```python
from build123d import *

# Parameters (mm, degrees)
CONECUT_DEPTH      = 53.387999569
CONECUT_DEPTH_BACK = 53.387999569


with BuildPart() as part:
    # Body: sweep along a path in PathSke
    with BuildLine(Plane.XY) as body_path:
        Line((45, 4.75), (0, 4.75))
        ThreePointArc((0, 4.75), (-1.846620522, 5.148259898), (-3.364941176, 6.272235294))
        ThreePointArc((-3.364941176, 6.272235294), (-20, 0), (-3.364941176, -6.272235294))
        ThreePointArc((-3.364941176, -6.272235294), (-1.846620522, -5.148259898), (0, -4.75))
        Line((0, -4.75), (51.3, -4.75))
    # SectionSke → Body (sweep)
    with BuildSketch(Plane(origin=(45, 0, 0), x_dir=(0, 0, -1), z_dir=(1, 0, 0))):
        with BuildLine():
            Line((-4.749999579, 0.002), (4.749999579, 0.002))
            ThreePointArc((4.749999579, 0.002), (0, 4.75), (-4.749999579, 0.002))
        make_face()
    sweep(path=body_path.line)

    # ConeCutSke → ConeCut (cut, two sides: drawn at the far end of the back side and taken through both)
    with BuildSketch(Plane.XY.offset(-CONECUT_DEPTH_BACK)):
        Polygon((45, 2.376), (41.603808574, 4.76), (51.31, 4.76), (51.31, -4.76), (47.903808574, -4.76), (51.3, -2.376), (47.898206914, 0), (41.598206914, 0), align=None)
    extrude(amount=CONECUT_DEPTH + CONECUT_DEPTH_BACK, mode=Mode.SUBTRACT)


solid = part.part
```
Design review of the part built by this model. Coordinates are the model's own, in mm. A direction names the side the tool comes from. Round coordinates to 2 decimals unless told otherwise and drop trailing zeros. Order: outer loops, then holes, each group sorted by start corner. A loop starts at its lowest first (then second) coordinate and runs counter-clockwise, first axis right, second up. Notation, with made-up numbers: (88, -27) - (140, -27) arc R26 ccw to (140, 6) - close; hole circle Ø1 at (54, 28). An arc over 180 degrees is marked (long way). Return JSON: item names as keys, results as strings.
Q1. Machinability: for faces 1 (the cylindrical face through (-15.25, 0.16, -0.07)), 2 (the cylindrical face through (26.01, -4.75, 0.1)), 3 (the cylindrical face through (22.18, 4.75, 0.1)), which of the approach directions +Z, -Z, +X, -X, +Y, -Y give a long, thin tool a straight path to every point of the face, cutting with its end or side? Answer none if there is none.
Computed values:
{"face 1": "+Z, -Z", "face 2": "+X, -Y", "face 3": "+X, +Y"}
Q2. Consider section B-B on x = 43.5. Write out the cut boundary in (y, z), plus the area to 3 significant figures.
Computed values:
{"outline": "(0, -4.75) - (0, 4.75) arc R4.75 ccw to start; (1.33, -4.56) arc R4.75 ccw to (3.43, -3.29) - (3.43, 3.29) arc R4.75 ccw to (1.33, 4.56) - close", "area": "52.4 mm2"}
Q3. Consider section A-A on z = 0. Write out the cut boundary in (x, y), plus the area to 3 significant figures.
Computed values:
{"outline": "(-6.93, -3.14) arc R4.75 cw (long way) to (-6.93, 3.14) arc R9.23 ccw to (0, 0) - (41.6, 0) - (45, 2.38) - (41.62, 4.75) - (0, 4.75) arc R4.48 cw to (-3.36, 6.27) arc R9.5 ccw (long way) to (-3.36, -6.27) arc R4.48 cw to (0, -4.75) - (47.92, -4.75) - (51.3, -2.38) - (47.9, 0) - (0, 0) arc R9.23 ccw to start", "area": "660 mm2"}
Q4. For pin 1 Ø1 at (x, y) = (-0.5, -2) entering from +Z; pin 2 Ø3 at (x, z) = (9.5, 2) entering from +Y; pin 3 Ø1.5 at (y, z) = (-3.5, -1) entering from +X, all flat-tipped, find the tip position at first contact; note any pin that passes through.
Computed values:
{"pin 1": "stops at z = 4.51", "pin 2": "stops at y = 4.72", "pin 3": "stops at x = 50.77"}
Q5. Wall thickness on L1, parallel to Y at x = -12, z = 0.75; L2, parallel to X at y = -2.5, z = -4; L3, parallel to X at y = -1, z = 1.5: over which ranges is each line inside the solid? List them lowest first. Write a range as [from, to].
Computed values:
{"L1": "y = [-9.32, -4.51], [4.51, 9.32]", "L2": "x = [-17.37, -14.54], [-6.31, 51.12]", "L3": "x = [-19.7, -15.15], [-4.17, 49.33]"}
Q6. The part is to be moulded in two halves that separate along Y. For faces 4 (the cylindrical face through (-3.75, 0.8, -0.07)), 5 (the flat face through (43.71, 3.28, -0.06)), 6 (the flat face through (49.961, -3.316, -0.058)), say which applies: pulls with the +Y half, pulls with the -Y half, needs draft (parallel to the pull), parting line crosses it, or undercut.
Computed values:
{"face 4": "undercut", "face 5": "pulls with the +Y half", "face 6": "pulls with the -Y half"}
Q7. Consider section D-D on z = 3.5. Write out the cut boundary in (x, y), plus the area to 3 significant figures.
Computed values:
{"outline": "(-6.93, -3.14) arc R4.75 cw (long way) to (-6.93, 3.14) arc R9.23 ccw to (0, 0) - (41.6, 0) - (45, 2.38) - (43.81, 3.21) - (0, 3.21) arc R6.02 cw to (-4.52, 5.26) arc R7.96 ccw (long way) to (-4.52, -5.26) arc R6.02 cw to (0, -3.21) - (50.11, -3.21) - (51.3, -2.38) - (47.9, 0) - (0, 0) arc R9.23 ccw to start", "area": "440 mm2"}
